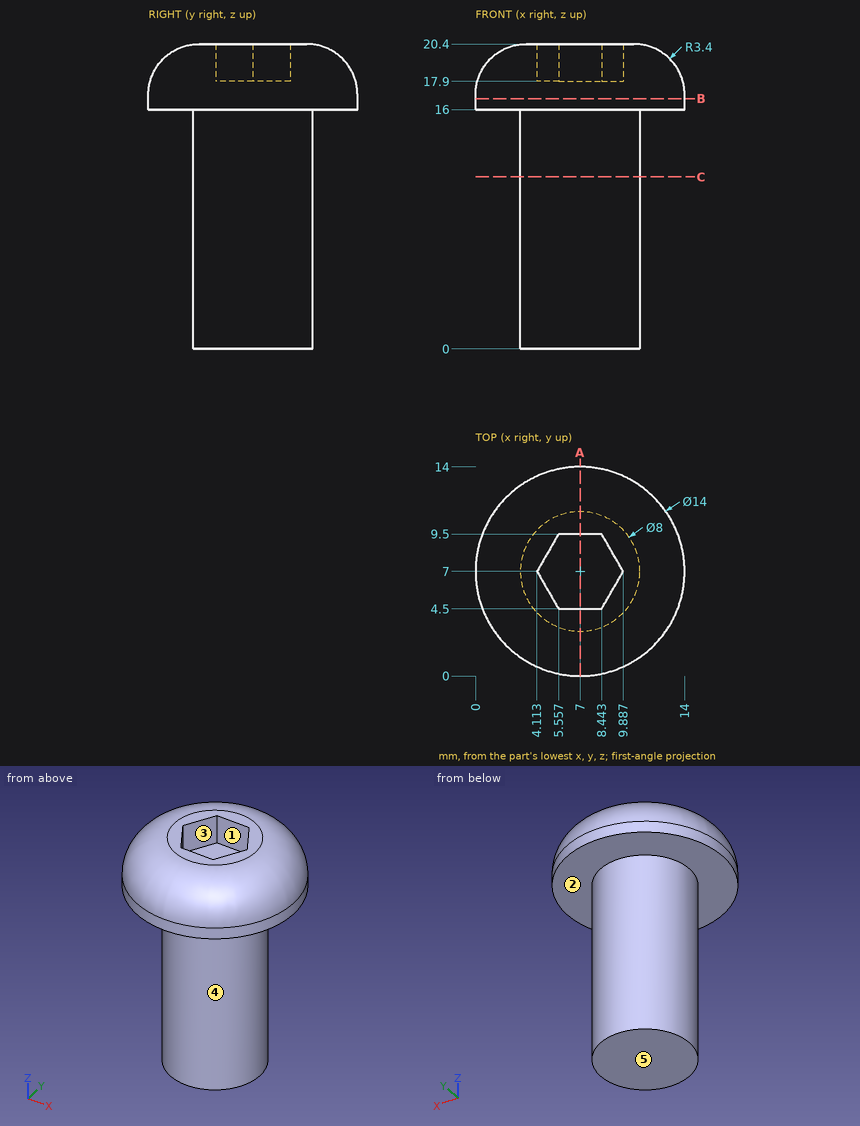
Study the drawing (mm; zero at the part's minimum x, y, z) and answer. A direction names the side the tool comes from. Give positions to 0.01 mm unless a question says otherwise; leave off trailing zeros. Write each loop counter-clockwise with the first axis right and the second up, starting at its lowest first coordinate (ties: lowest second). Pieces come first, ordered by that corner, then holes. Notation, with made-up numbers: (-14, -23.5) -> (38, -23.5) arc R24 ccw to (38, -6.5) -> close; hole circle Ø2 at (7.5, 59.5). An arc over 180 degrees is marked (long way). Write item = value, one per line. Start each with the question number.
1) The part is cut by section C-C, the plane z = 11.5. Determine the outline of the cut face in (x, y).
2) Each of these flat-tipped pins is pushed along its axis until it touches: pin 1 (4 mm diameter, centred on x = 4.5, y = 6.5, fed in from -Z); pin 2 (2 mm diameter, centred on y = 4.5, z = 8.5, fed in from +X); pin 3 (4 mm diameter, centred on x = 4.5, z = 18, fed in from +Y); pin 4 (3 mm diameter, centred on x = 1.5, y = 8, fed in from +Z) (1 decimal). Where does it stop, or does it pass through?
3) Which of the six approach directions +Z, -Z, +X, -X, +Y, -Y give full straight-line access (tool end or side, diameter ignored) to the marked faces 1 and 2?
4) Determine the mould class of the marked faces 3, 4 and 5 for opening direction X: +X half, -X half, draft (parallel to the pull), parting line (faces both ways), or undercut.
5) The part is cut by section A-A, the plane x = 7. Determine the outline of the cut face in (y, z), and give its area (3 significant figures).
6) Straight lines are drawn through the part: line 1 along X through (y, z) = (10, 15.75) (1 decimal); line 2 along Y through (x, z) = (7.75, 11); line 3 along Z through (x, y) = (3.75, 2) (1 decimal). For each, find the intervals that lie inside material, in ascending order.
7) The part is cut by section B-B, the plane z = 16.75. Determine the outline of the cut face in (x, y), and give its area (3 significant figures).
Solutions:
q1.outline = circle Ø8 at (7, 7)
q2.pin_1 = 0
q2.pin_2 = 10.71
q2.pin_3 = 13.96
q2.pin_4 = 20.4
q3.face_1 = +Z
q3.face_2 = -Z
q4.face_3 = undercut
q4.face_4 = parting line
q4.face_5 = draft
q5.outline = (0, 16) -> (3, 16) -> (3, 0) -> (11, 0) -> (11, 16) -> (14, 16) -> (14, 17) arc R3.4 ccw to (10.6, 20.4) -> (9.5, 20.4) -> (9.5, 17.9) -> (4.5, 17.9) -> (4.5, 20.4) -> (3.4, 20.4) arc R3.4 ccw to (0, 17) -> close
q5.area = 172 mm²
q6.line_1 = 4.4 to 9.6
q6.line_2 = 3.07 to 10.93
q6.line_3 = 16 to 19.4
q7.outline = circle Ø14 at (7, 7)
q7.area = 154 mm²
